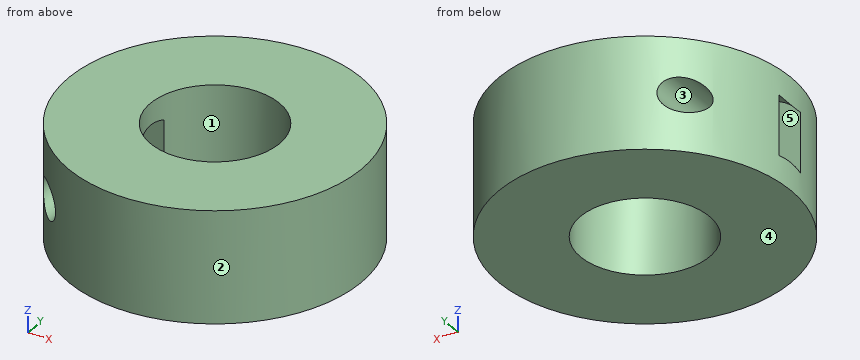
from build123d import *

# Parameters (mm, degrees)
F0_R          = 34
F0_R_2        = 15
F1_DEPTH      = 26
F2_R          = 12
F3_DEPTH      = 4
F3_DEPTH_BACK = 4
F4_R          = 4
F5_DEPTH      = 34.0010001
F5_DEPTH_BACK = 34.0010001


with BuildPart() as f1:
    # F0 (on Top) → F1 (new body)
    with BuildSketch(Plane.XY):
        Circle(F0_R)
        Circle(F0_R_2, mode=Mode.SUBTRACT)
    extrude(amount=F1_DEPTH)

    # F2 (on Front) → F3 (cut, two sides)
    with BuildSketch(Plane.XZ) as f3_sk:
        with Locations((-24, 13)):
            Circle(F2_R)
    extrude(amount=-F3_DEPTH, mode=Mode.SUBTRACT)
    extrude(f3_sk.sketch, amount=F3_DEPTH_BACK, mode=Mode.SUBTRACT)

    # F4 (on Front) → F5 (cut, two sides)
    with BuildSketch(Plane.XZ) as f5_sk:
        with Locations((-24, 13)):
            Circle(F4_R)
    extrude(amount=F5_DEPTH, mode=Mode.SUBTRACT)
    extrude(f5_sk.sketch, amount=-F5_DEPTH_BACK, mode=Mode.SUBTRACT)


solid = f1.part
Work out the finished part from the listing and answer in its coordinate system (mm). Face numbers are marked on the shaded views. A direction names the side the tool comes from. Give positions to 0.01 mm unless a question says otherwise; leave off trailing zeros. Loops run counter-clockwise (first coordinate to the right, second up) from the corner with the lowest first, then second, coordinate; pieces in that order, holes last. Notation, with made-up numbers: (-23, 52) - (32, 52) arc R20 ccw to (32, 83) - close; hole circle Ø11 at (35, 76). An arc over 180 degrees is marked (long way). Answer in a Markdown table with one row per item. Add a question column.
Q1. The part is cut by section B-B (x = 0). Determine the outline of the cut face in (y, z).
Q2. A tool of negligible diameter and unlimited length cuts with its end or side. For the marked faces 4 and 5, from which of +Z, -Z, +X, -X, +Y, -Y can it reach the whole face along a straight path? Write none if from no direction.
Q3. Determine the mould class of the marked faces 1, 2 and 3 for opening direction Y: released by +Y, released by -Y, zero draft, split by the parting line, or undercut.
Q4. The part is cut by section A-A (y = -9). Determine the outline of the cut face in (x, z), and give its area (3 significant figures).
Q5. The part is cut by section D-D (y = 0). Determine the outline of the cut face in (x, z).
Q6. Consider line 1 along Z through (x, y) = (-24, 11.75); line 2 along Y through (x, z) = (0, 14); line 3 along X through (y, z) = (-11, 13). Determine where each line is inside the solid, lowest interval first.
Q7. Each of these flat-tipped pins is pushed along its axis until it touches: P1, Ø10.5, axis at x = -24, z = 13, coming from the +Y side; P2, Ø12, axis at x = -23, z = 20.5, coming from the +Y side; P3, Ø1.5, axis at y = 24, z = 11, coming from the +X side; P4, Ø18, axis at x = 0, y = 0, coming from the +Z side. Where does it stop, or does it pass through?
Q8. The part is cut by section C-C (z = 14). Determine the outline of the cut face in (x, y), and give its area (3 significant figures).
Solution:
| question | item | result |
|---|---|---|
| 1 | outline | (-34, 0) - (-15, 0) - (-15, 26) - (-34, 26) - close; (15, 0) - (34, 0) - (34, 26) - (15, 26) - close |
| 2 | face 4 | -Z, +X, -X, +Y, -Y |
| 2 | face 5 | none |
| 3 | face 1 | undercut |
| 3 | face 2 | split by the parting line |
| 3 | face 3 | zero draft |
| 4 | outline | (-32.79, 0) - (-12, 0) - (-12, 26) - (-32.79, 26) - close; (12, 0) - (32.79, 0) - (32.79, 26) - (12, 26) - close; hole circle Ø8 at (-24, 13) |
| 4 | area | 1,030 mm² |
| 5 | outline | (-34, 0) - (-15, 0) - (-15, 5.06) arc R12 cw to (-34, 6.37) - close; (-34, 19.63) arc R12 cw to (-15, 20.94) - (-15, 26) - (-34, 26) - close; (15, 0) - (34, 0) - (34, 26) - (15, 26) - close |
| 6 | line 1 | z = 0 to 9, 17 to 26 |
| 6 | line 2 | y = -34 to -15, 15 to 34 |
| 6 | line 3 | x = -32.17 to -28, -20 to -10.2, 10.2 to 32.17 |
| 7 | P1 | stops at y = 28.36 |
| 7 | P2 | stops at y = 29.44 |
| 7 | P3 | stops at x = 24.81 |
| 7 | P4 | passes through |
| 8 | outline | (-33.76, -4) arc R34 ccw to (-27.87, -19.47) - (-27.87, -4) - close; (-33.76, 4) - (-27.87, 4) - (-27.87, 19.47) arc R34 ccw to start; (-20.13, -27.4) arc R34 ccw (long way) to (-20.13, 27.4) - (-20.13, 4) - (-14.46, 4) arc R15 cw (long way) to (-14.46, -4) - (-20.13, -4) - close |
| 8 | area | 2,460 mm² |
